Verification items for this drawing (mm, ordinates from the low corner). A direction names the side the tool comes from. Coordinates: 2 decimals unless noted, no trailing zeros. Order: outer loops, then holes, each group sorted by start corner. A loop starts at its lowest first (then second) coordinate and runs counter-clockwise, first axis right, second up. Notation, with made-up numbers: M -36,74.5 L -23,74.5 A28 ccw -23,93.5 Z; hole C 35.25,52.5 d9. An arc over 180 degrees is marked long. Write item = value, one per line.
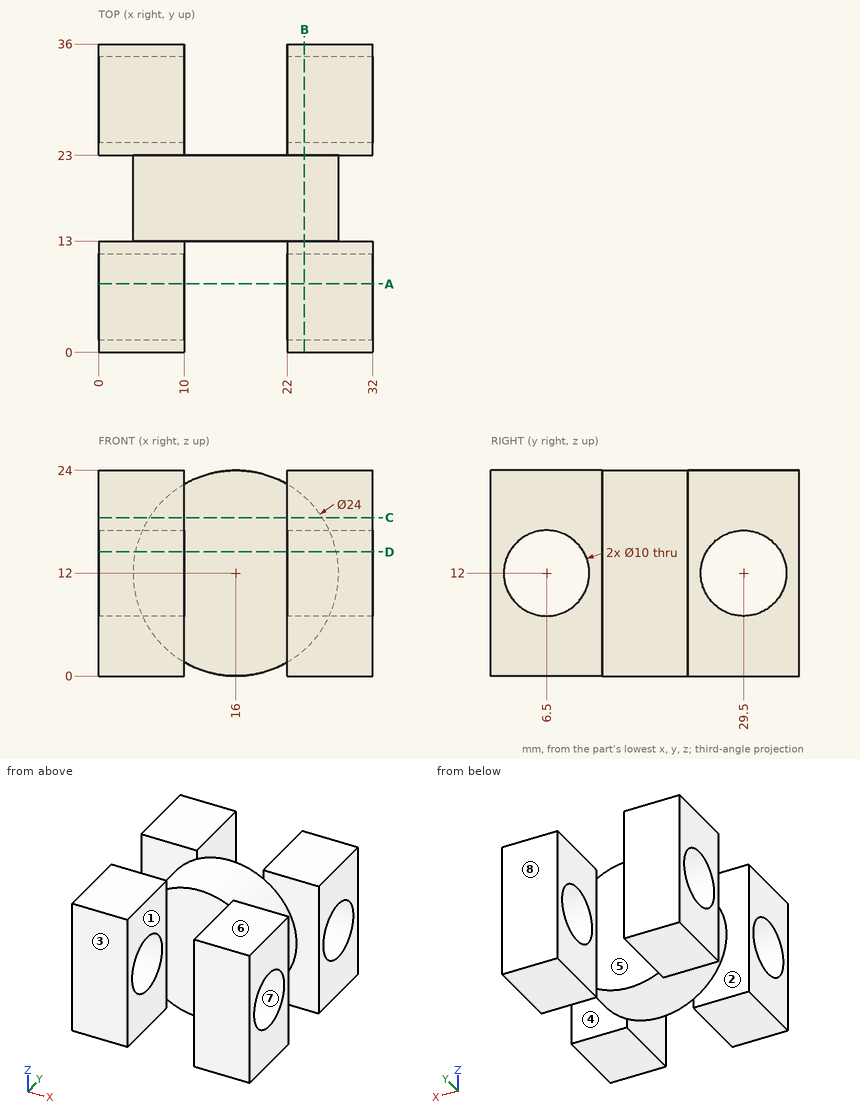
Item 1: Sectioned sample at D-D, the plane z = 14.5. Give the number of separate pieces and of enclosed holes in the cut face, then the cut area to 3 significant figures.
Report:
separate_pieces = 5
enclosed_holes = 0
area = 408 mm^2
Item 2: Sectioned sample at B-B, the plane x = 24. Enter the section's corners in (y, z), then the cut area to 3 significant figures.
Report:
outline = M 0,0 L 13,0 L 13,3.06 L 23,3.06 L 23,0 L 36,0 L 36,24 L 23,24 L 23,20.94 L 13,20.94 L 13,24 L 0,24 Z; hole C 6.5,12 d10; hole C 29.5,12 d10
area = 646 mm^2
Item 3: Tool access check on the marked faces 1, 2, 3, 4 and 5. Record the directions out of +Z, -Z, +X, -X, +Y, -Y that give a thin tool (end or side, any length) a straight path to the whole face; none if there is none.
Report:
face_1 = +Z, -Z, -Y
face_2 = -X
face_3 = +Z, -Z, +X, -X, -Y
face_4 = +X
face_5 = +Z, -Z, +Y
Item 4: Scan lines: L1, parallel to Y at x = 6.5, z = 12; L2, parallel to Y at x = 29.25, z = 12; L3, parallel to X at y = 34.5, z = 10.5. Record each from-to range of solid material in increasing order. Write a range as from..to.
Report:
L1 = 0..1.5, 11.5..24.5, 34.5..36
L2 = 0..1.5, 11.5..13, 23..24.5, 34.5..36
L3 = 0..10, 22..32
Item 5: Release check for a two-part mould opening along Z. For the marked faces 6, 7 and 8 record: pulls with the +Z half, pulls with the -Z half, needs draft (parallel to the pull), parting line crosses it, or undercut.
Report:
face_6 = pulls with the +Z half
face_7 = undercut
face_8 = needs draft
Item 6: Sectioned sample at A-A, the plane y = 8. Enter the section's corners in (x, z), then the cut area to 3 significant figures.
Report:
outline = M 0,0 L 10,0 L 10,7.23 L 0,7.23 Z; M 0,16.77 L 10,16.77 L 10,24 L 0,24 Z; M 22,0 L 32,0 L 32,7.23 L 22,7.23 Z; M 22,16.77 L 32,16.77 L 32,24 L 22,24 Z
area = 289 mm^2
Item 7: Sectioned sample at C-C, the plane z = 18.5. Enter the section's corners in (x, y), then the cut area to 3 significant figures.
Report:
outline = M 0,0 L 10,0 L 10,13 L 22,13 L 22,0 L 32,0 L 32,13 L 26.09,13 L 26.09,23 L 32,23 L 32,36 L 22,36 L 22,23 L 10,23 L 10,36 L 0,36 L 0,23 L 5.91,23 L 5.91,13 L 0,13 Z
area = 722 mm^2
Item 8: Gauge pin test, flat ends, axial feed: pin 1 (13 mm diameter, centred on y = 29.5, z = 12, fed in from -X); pin 2 (3.5 mm diameter, centred on x = 15, z = 7, fed in from +Y); pin 3 (6 mm diameter, centred on x = 17.5, z = 10, fed in from -Y). Record the tip position at first contact, or that the pin passes through.
Report:
pin_1 = 0
pin_2 = 23
pin_3 = 13
